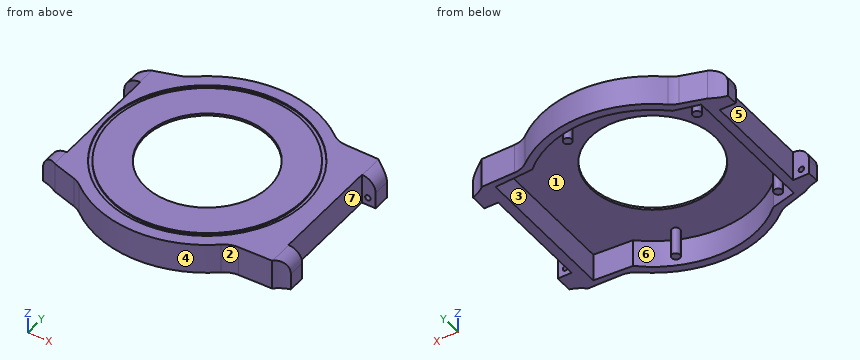
from build123d import *

# Parameters (mm, degrees)
PAD_DEPTH       = 6.5
POCKET_DEPTH    = 6
SKETCH002_R     = 13.5
POCKET001_DEPTH = 1
SKETCH003_W     = 5.4
SKETCH003_H     = 6.5
PAD001_DEPTH    = 3
POCKET002_DEPTH = 10
SKETCH008_R     = 0.6
POCKET003_DEPTH = 2
SKETCH009_R     = 0.6
POCKET004_DEPTH = 2
FILLET_R        = 2.9
FILLET001_R     = 2.9
FILLET002_R     = 5
FILLET003_R     = 5
FILLET004_R     = 5
FILLET005_R     = 5
SKETCH010_W     = 3.95
SKETCH010_H     = 6.5
PAD002_DEPTH    = 3.5
POCKET005_DEPTH = 10
SKETCH012_R     = 0.6
POCKET006_DEPTH = 2
SKETCH013_R     = 0.6
POCKET007_DEPTH = 2
FILLET006_R     = 3.4
FILLET007_R     = 3.4
SKETCH014_R     = 21.6
SKETCH014_R_2   = 20.8
POCKET008_DEPTH = 0.3
SKETCH015_R     = 0.9
PAD003_DEPTH    = 6


with BuildPart() as part:
    # Sketch → Pad (new body)
    with BuildSketch(Plane.XY):
        with BuildLine():
            Line((-22.501992, 16), (-22.501992, -16))
            Line((-22.501992, -16), (-16.285883, -17.9))
            ThreePointArc((-16.285883, -17.9), (0.22069, -24.198994), (16.609636, -17.6))
            Line((16.609636, -17.6), (25.608386, -17.45))
            Line((25.608386, 17.45), (25.608386, -17.45))
            Line((16.609636, 17.6), (25.608386, 17.45))
            ThreePointArc((16.609636, 17.6), (0.22069, 24.198994), (-16.285883, 17.9))
            Line((-22.501992, 16), (-16.285883, 17.9))
        make_face()
    extrude(amount=PAD_DEPTH)

    # Sketch001 → Pocket (cut)
    with BuildSketch(Plane.XY):
        with BuildLine():
            Line((-15.242949, 16.55), (-20.574694, 15.2))
            Line((-20.574694, 15.2), (-20.574694, -15.2))
            Line((-20.574694, -15.2), (-15.242949, -16.55))
            ThreePointArc((-15.242949, -16.55), (0, -22.5), (15.242949, -16.55))
            Line((15.242949, -16.55), (23.527875, -16.05))
            Line((23.527875, 16.05), (23.527875, -16.05))
            Line((15.242949, 16.55), (23.527875, 16.05))
            ThreePointArc((15.242949, 16.55), (0, 22.5), (-15.242949, 16.55))
        make_face()
    extrude(amount=POCKET_DEPTH, mode=Mode.SUBTRACT)

    # Sketch002 (on Face19 of Pocket) → Pocket001 (cut)
    with BuildSketch(Plane(origin=(0, 0, 6), x_dir=(1, 0, 0), z_dir=(0, 0, -1))):
        Circle(SKETCH002_R)
    extrude(amount=-POCKET001_DEPTH, mode=Mode.SUBTRACT)

    # Sketch003 (on Face6 of Pocket001) → Pad001 (join)
    with BuildSketch(Plane.YZ.offset(25.608386)):
        with Locations((-14.75, 3.25)):
            Rectangle(SKETCH003_W, SKETCH003_H)
        with Locations((14.75, 3.25)):
            Rectangle(SKETCH003_W, SKETCH003_H)
    extrude(amount=PAD001_DEPTH)

    # Sketch006 → Pocket002 (cut)
    with BuildSketch(Plane.XY.offset(6.5)):
        with BuildLine():
            ThreePointArc((25.608386, 17.45), (27.01354, 16.442644), (28.608386, 15.775042))
            Line((28.608386, 17.45), (28.608386, 15.775042))
            Line((28.608386, 17.45), (25.608386, 17.45))
        make_face()
        with BuildLine():
            ThreePointArc((28.608386, -15.775042), (27.01354, -16.442644), (25.608386, -17.45))
            Line((28.608386, -17.45), (25.608386, -17.45))
            Line((28.608386, -15.775042), (28.608386, -17.45))
        make_face()
    extrude(amount=-POCKET002_DEPTH, mode=Mode.SUBTRACT)

    # Sketch008 (on Face27 of Pocket002) → Pocket003 (cut)
    with BuildSketch(Plane(origin=(0, -12.05, 0), x_dir=(-1, 0, 0), z_dir=(0, 1, 0))):
        with Locations((-26.908386, 1.7)):
            Circle(SKETCH008_R)
    extrude(amount=-POCKET003_DEPTH, mode=Mode.SUBTRACT)

    # Sketch009 (on Face26 of Pocket003) → Pocket004 (cut)
    with BuildSketch(Plane.XZ.offset(-12.05)):
        with Locations((26.908386, 1.7)):
            Circle(SKETCH009_R)
    extrude(amount=-POCKET004_DEPTH, mode=Mode.SUBTRACT)

    # Fillet
    fillet_edges = [part.edges().sort_by_distance(p)[0] for p in [
        (28.608386, -13.912521, 6.5),
    ]]
    fillet(fillet_edges, radius=FILLET_R)

    # Fillet001
    fillet001_edges = [part.edges().sort_by_distance(p)[0] for p in [
        (28.608386, 13.912521, 6.5),
    ]]
    fillet(fillet001_edges, radius=FILLET001_R)

    # Fillet002
    fillet002_edges = [part.edges().sort_by_distance(p)[0] for p in [
        (16.609636, -17.6, 3.25),
    ]]
    fillet(fillet002_edges, radius=FILLET002_R)

    # Fillet003
    fillet003_edges = [part.edges().sort_by_distance(p)[0] for p in [
        (16.609636, 17.6, 3.25),
    ]]
    fillet(fillet003_edges, radius=FILLET003_R)

    # Fillet004
    fillet004_edges = [part.edges().sort_by_distance(p)[0] for p in [
        (-16.285883, -17.9, 3.25),
    ]]
    fillet(fillet004_edges, radius=FILLET004_R)

    # Fillet005
    fillet005_edges = [part.edges().sort_by_distance(p)[0] for p in [
        (-16.285883, 17.9, 3.25),
    ]]
    fillet(fillet005_edges, radius=FILLET005_R)

    # Sketch010 (on Face4 of Fillet005) → Pad002 (join)
    with BuildSketch(Plane(origin=(-22.501992, 0, 0), x_dir=(0, -1, 0), z_dir=(-1, 0, 0))):
        with Locations((-14.025, 3.25)):
            Rectangle(SKETCH010_W, SKETCH010_H)
        with Locations((14.025, 3.25)):
            Rectangle(SKETCH010_W, SKETCH010_H)
    extrude(amount=PAD002_DEPTH)

    # Sketch011 (on Face6 of Pad002) → Pocket005 (cut)
    with BuildSketch(Plane.XY.offset(6.5)):
        with BuildLine():
            ThreePointArc((-26.001992, 14.6), (-24.192608, 15.15154), (-22.501992, 16))
            Line((-22.501992, 16), (-26.001992, 16))
            Line((-26.001992, 16), (-26.001992, 14.6))
        make_face()
        with BuildLine():
            ThreePointArc((-22.501992, -16), (-24.192608, -15.15154), (-26.001992, -14.6))
            Line((-26.001992, -14.6), (-26.001992, -16))
            Line((-26.001992, -16), (-22.501992, -16))
        make_face()
    extrude(amount=-POCKET005_DEPTH, mode=Mode.SUBTRACT)

    # Sketch012 (on Face23 of Pocket005) → Pocket006 (cut)
    with BuildSketch(Plane(origin=(0, -12.05, 0), x_dir=(-1, 0, 0), z_dir=(0, 1, 0))):
        with Locations((24.301992, 1.7)):
            Circle(SKETCH012_R)
    extrude(amount=-POCKET006_DEPTH, mode=Mode.SUBTRACT)

    # Sketch013 (on Face21 of Pocket006) → Pocket007 (cut)
    with BuildSketch(Plane.XZ.offset(-12.05)):
        with Locations((-24.301992, 1.7)):
            Circle(SKETCH013_R)
    extrude(amount=-POCKET007_DEPTH, mode=Mode.SUBTRACT)

    # Fillet006
    fillet006_edges = [part.edges().sort_by_distance(p)[0] for p in [
        (-26.001992, 13.325, 6.5),
    ]]
    fillet(fillet006_edges, radius=FILLET006_R)

    # Fillet007
    fillet007_edges = [part.edges().sort_by_distance(p)[0] for p in [
        (-26.001992, -13.325, 6.5),
    ]]
    fillet(fillet007_edges, radius=FILLET007_R)

    # Sketch014 (on Face4 of Fillet007) → Pocket008 (cut)
    with BuildSketch(Plane.XY.offset(6.5)):
        Circle(SKETCH014_R)
        Circle(SKETCH014_R_2, mode=Mode.SUBTRACT)
    extrude(amount=-POCKET008_DEPTH, mode=Mode.SUBTRACT)

    # Sketch015 (on Face55 of Pocket008) → Pad003 (join)
    with BuildSketch(Plane(origin=(0, 0, 6), x_dir=(1, 0, 0), z_dir=(0, 0, -1))):
        with Locations((-18.42, 13.32)):
            Circle(SKETCH015_R)
        with Locations((-18.42, -13.32)):
            Circle(SKETCH015_R)
        with Locations((7.27, 18.56)):
            Circle(SKETCH015_R)
        with Locations((5.37, -19.79)):
            Circle(SKETCH015_R)
    extrude(amount=PAD003_DEPTH)


solid = part.part
Source: CAD feature listing. Evaluate the final solid. Frame: model axes, mm. Face numbers are marked on the shaded views. A direction names the side the tool comes from. Round coordinates to 2 decimals unless told otherwise and drop trailing zeros. Loops run counter-clockwise (first coordinate to the right, second up) from the corner with the lowest first, then second, coordinate; pieces in that order, holes last. Notation, with made-up numbers: M -5.75,17.5 L 16.25,17.5 A27 ccw 16.25,37.5 Z; hole C 53,47 d6. An arc over 180 degrees is marked long. Answer as CSV lines item,"result".
Q1. Reachability of the marked faces 5, 6 and 7 from +Z, -Z, +X, -X, +Y, -Y: full face, straight path, thin tool, end or side. Return the list, or none.
Verdict:
face 5,"+Z, -Z, -X"
face 6,"-Z"
face 7,"+Z, -Z, +X"
Q2. Cut plane A-A (x = 0). Return the cut outline in (y, z).
Verdict:
outline,"M -24.2,0 L -22.5,0 L -22.5,6 L -13.5,6 L -13.5,6.5 L -20.8,6.5 L -20.8,6.2 L -21.6,6.2 L -21.6,6.5 L -24.2,6.5 Z; M 13.5,6 L 22.5,6 L 22.5,0 L 24.2,0 L 24.2,6.5 L 21.6,6.5 L 21.6,6.2 L 20.8,6.2 L 20.8,6.5 L 13.5,6.5 Z"
Q3. Cut plane B-B (y = 10). Return the cut outline in (x, z), plus the area to 3 significant figures.
Verdict:
outline,"M -22.5,0 L -20.57,0 L -20.57,6 L -9.07,6 L -9.07,6.5 L -18.24,6.5 L -18.24,6.2 L -19.15,6.2 L -19.15,6.5 L -22.5,6.5 Z; M 9.07,6 L 23.53,6 L 23.53,0 L 25.61,0 L 25.61,6.5 L 19.15,6.5 L 19.15,6.2 L 18.24,6.2 L 18.24,6.5 L 9.07,6.5 Z"
area,"38.5 mm^2"
Q4. Cut plane D-D (x = 7.27). Return the cut outline in (y, z).
Verdict:
outline,"M -23.08,0 L -21.29,0 L -21.29,6 L -19.46,6 L -19.46,0 L -17.66,0 L -17.66,6 L -11.38,6 L -11.38,6.5 L -19.49,6.5 L -19.49,6.2 L -20.34,6.2 L -20.34,6.5 L -23.08,6.5 Z; M 11.38,6 L 21.29,6 L 21.29,0 L 23.08,0 L 23.08,6.5 L 20.34,6.5 L 20.34,6.2 L 19.49,6.2 L 19.49,6.5 L 11.38,6.5 Z"
Q5. Pull-direction query (X, two-part tool) for the marked faces 1, 2, 3 and 4; classes: +X half, -X half, draft (parallel to the pull), parting line (faces both ways), or undercut.
Verdict:
face 1,"undercut"
face 2,"+X half"
face 3,"undercut"
face 4,"parting line"
Q6. Cut plane C-C (z = 4.75). Count the separate pieces of the cut face and the enclosed holes in it, plus the area to 3 significant figures.
Verdict:
separate pieces,"5"
enclosed holes,"1"
area,"343 mm^2"
Q7. Contact query for flat-ended pins moving along their axis: pin 1 (2 mm diameter, centred on y = 3, z = 2.5, fed in from +X); pin 2 (3 mm diameter, centred on y = -4.5, z = 4, fed in from -X); pin 3 (1.8 mm diameter, centred on x = -24, z = 3.5, fed in from +Y). Output: stop coordinate, or through.
Verdict:
pin 1,"stops at x = 25.61"
pin 2,"stops at x = -22.5"
pin 3,"stops at y = 15.66"
Q8. Line query: line 1 along X through (y, z) = (1, 1.5); line 2 along X through (y, z) = (-18.5, 2.25); line 3 along X through (y, z) = (-14, 3.5). Output: solid intervals per line, ascending.
Verdict:
line 1,"x = -22.5 to -20.57, 23.53 to 25.61"
line 2,"x = -15.6 to -12.81, 6.37 to 8.17, 12.81 to 15.62"
line 3,"x = -25.98 to -20.57, -19.01 to -17.83, 23.53 to 28.61"
